Work out the finished part from the listing and answer in its coordinate system (mm). Coordinates: 2 decimals unless noted, no trailing zeros. Order: outer loops, then holes, each group sorted by start corner. A loop starts at its lowest first (then second) coordinate and runs counter-clockwise, first axis right, second up. Notation, with made-up numbers: M 87,85 L 132,85 A18 cw 132,116 Z; hole C 7,79 d3. An arc over 180 degrees is marked long. Answer in a Markdown table with one row per item. Add a question column.
Item 1: Flat-ended cylindrical pins translate along their axes: pin 1 Ø9 at (x, y) = (0, 0) entering from -Z; pin 2 Ø3 at (x, y) = (-15, 16) entering from -Z; pin 3 Ø1 at (y, z) = (-14.5, 2) entering from +X. Find the tip coordinate at first contact, or state that the pin passes through.
Item 2: The part is cut by section C-C (z = 0.5). Write down the section's boundary in (x, y).
Item 3: Consider line 1 (Y direction, x = 0, z = 0.75); line 2 (Y direction, x = 0, z = 1.05); line 3 (X direction, y = -2, z = 1.2). Determine where each line is inside the solid, lowest interval first. Write a range as from..to.
Item 4: The mould has two halves that part along X. Classify faces 1 (the face through (-7.493, 0.33, 0.986)), 2 (the face through (-4.769, -21.477, 1.493)), 3 (the face through (9, 0, 0)): released by +X, released by -X, zero draft, split by the parting line, or undercut.
Item 5: The part is cut by section A-A (y = 0). Write down the section's boundary in (x, z), then the cut area to 3 significant figures.
from build123d import *

# Parameters (mm, degrees)
SKETCH_1_R                  = 22
SKETCH_1_R_2                = 7.5
EXTRUDE_1_DEPTH             = 2
CHAMFER_1_SIZE              = 1
HOLE_WIZARD_M4_1_AT_2_COUNT = 2
HOLE_WIZARD_M4_1_AT_2_PITCH = 28
HOLE_WIZARD_M4_1_AT_3_COUNT = 2
HOLE_WIZARD_M4_1_AT_3_PITCH = 19.798989873
HOLE_WIZARD_M4_1_AT_4_COUNT = 2
HOLE_WIZARD_M4_1_AT_4_PITCH = 19.798989873


with BuildPart() as part:
    # 草图1 → 凸台-拉伸1 (new body)
    with BuildSketch(Plane.XY):
        Circle(SKETCH_1_R)
        Circle(SKETCH_1_R_2, mode=Mode.SUBTRACT)
    extrude(amount=EXTRUDE_1_DEPTH)

    # 倒角1
    chamfer_1_edges = [part.edges().sort_by_distance(p)[0] for p in [
        (-22, 0, 0),
    ]]
    chamfer(chamfer_1_edges, length=CHAMFER_1_SIZE)

    # 草图2 → M4 六角凹锥坑螺钉的锥形沉头孔1 (revolve, cut)
    with BuildSketch(Plane(origin=(0, 14, 2), x_dir=(0, -1, 0), z_dir=(1, 0, 0))):
        Polygon((0, 0), (0, 2), (2.25, 2), (2.25, 2.23), (4.48, 0), align=None)
    hole_wizard_m4_1 = revolve(axis=Axis((0, 14, 8.35), (0, 0, -1)), mode=Mode.SUBTRACT)

    # M4 六角凹锥坑螺钉的锥形沉头孔1 at 2: M4 六角凹锥坑螺钉的锥形沉头孔1 ×2
    with Locations(*[(0, -i * HOLE_WIZARD_M4_1_AT_2_PITCH, 0) for i in range(1, HOLE_WIZARD_M4_1_AT_2_COUNT)]):
        add(hole_wizard_m4_1, mode=Mode.SUBTRACT)

    # M4 六角凹锥坑螺钉的锥形沉头孔1 at 3: M4 六角凹锥坑螺钉的锥形沉头孔1 ×2
    with Locations(*[Vector(-0.7071067811865476, -0.7071067811865476, 0) * (i * HOLE_WIZARD_M4_1_AT_3_PITCH) for i in range(1, HOLE_WIZARD_M4_1_AT_3_COUNT)]):
        add(hole_wizard_m4_1, mode=Mode.SUBTRACT)

    # M4 六角凹锥坑螺钉的锥形沉头孔1 at 4: M4 六角凹锥坑螺钉的锥形沉头孔1 ×2
    with Locations(*[Vector(0.7071067811865475, -0.7071067811865476, 0) * (i * HOLE_WIZARD_M4_1_AT_4_PITCH) for i in range(1, HOLE_WIZARD_M4_1_AT_4_COUNT)]):
        add(hole_wizard_m4_1, mode=Mode.SUBTRACT)


solid = part.part
Reply:
| question | item | result |
|---|---|---|
| 1 | pin 1 | passes through |
| 1 | pin 2 | stops at z = 0 |
| 1 | pin 3 | stops at x = 16.97 |
| 2 | outline | C 0,0 d43; hole C -14,0 d5.96; hole C 0,0 d15; hole C 0,-14 d5.96; hole C 0,14 d5.96; hole C 14,0 d5.96 |
| 3 | line 1 | y = -21.75..-17.23, -10.77..-7.5, 7.5..10.77, 17.23..21.75 |
| 3 | line 2 | y = -22..-17.53, -10.47..-7.5, 7.5..10.47, 17.53..22 |
| 3 | line 3 | x = -21.91..-17.09, -10.91..-7.23, 7.23..10.91, 17.09..21.91 |
| 4 | face 1 | undercut |
| 4 | face 2 | split by the parting line |
| 4 | face 3 | zero draft |
| 5 | outline | M -22,1 L -21,0 L -16.48,0 L -18.48,2 L -22,2 Z; M -11.52,0 L -7.5,0 L -7.5,2 L -9.52,2 Z; M 7.5,0 L 11.52,0 L 9.52,2 L 7.5,2 Z; M 16.48,0 L 21,0 L 22,1 L 22,2 L 18.48,2 Z |
| 5 | area | 29.2 mm2 |
